Geometry: final body of the model. Coordinates: model frame, mm. Face numbers are marked on the shaded views. A direction names the side the tool comes from. Give positions to 0.01 mm unless a question says otherwise; leave off trailing zeros. Order: outer loops, then holes, each group sorted by start corner. A loop starts at its lowest first (then second) coordinate and runs counter-clockwise, first axis right, second up. Notation, with made-up numbers: (23, 53) -> (60, 53) arc R14 ccw to (60, 73) -> close; hole circle Ø5 at (18.25, 19). An arc over 180 degrees is marked (long way). Write item = value, one per line.
```python
from build123d import *

# Parameters (mm, degrees)
SKETCH1_W                      = 55
SKETCH1_H                      = 55
BOSS_EXTRUDE1_DEPTH            = 6.35
SKETCH2_W                      = 11.25
SKETCH2_H                      = 11.25
CUT_EXTRUDE1_DEPTH             = 7.35
SKETCH3_W                      = 14
SKETCH3_H                      = 8.5
CUT_EXTRUDE2_DEPTH             = 2
CBORE_FOR_M2_SHCS2_D           = 2.4
CBORE_FOR_M2_SHCS2_DEPTH       = 6.35
CBORE_FOR_M2_SHCS2_CBORE_D     = 4.4
CBORE_FOR_M2_SHCS2_CBORE_DEPTH = 2
SKETCH6_R                      = 3.25
BOSS_EXTRUDE2_DEPTH            = 5
CBORE_FOR_M2_SHCS1_D           = 2.4
CBORE_FOR_M2_SHCS1_CBORE_D     = 4.4
CBORE_FOR_M2_SHCS1_CBORE_DEPTH = 2
SKETCH13_R                     = 3.025
CUT_EXTRUDE4_DEPTH             = 1
CHAMFER1_SIZE                  = 2
SKETCH16_W                     = 10
SKETCH16_H                     = 10
BOSS_EXTRUDE3_DEPTH            = 6.35
SKETCH17_R                     = 2.55
CUT_EXTRUDE6_DEPTH             = 12.35
FILLET1_R                      = 5
FILLET2_R                      = 1
SKETCH18_R                     = 2.25
CUT_EXTRUDE7_DEPTH             = 1


with BuildPart() as part:
    # Sketch1 → Boss-Extrude1 (new body)
    with BuildSketch(Plane(origin=(0, 0, 0), x_dir=(1, 0, 0), z_dir=(0, 1, 0))):
        Rectangle(SKETCH1_W, SKETCH1_H)
    extrude(amount=BOSS_EXTRUDE1_DEPTH)

    # Sketch2 → Cut-Extrude1 (cut, through all)
    with BuildSketch(Plane(origin=(0, 6.35, 0), x_dir=(1, 0, 0), z_dir=(0, 1, 0))):
        Rectangle(SKETCH2_W, SKETCH2_H)
    extrude(amount=-CUT_EXTRUDE1_DEPTH, mode=Mode.SUBTRACT)

    # Sketch3 → Cut-Extrude2 (cut)
    with BuildSketch(Plane(origin=(0, 6.35, 0), x_dir=(1, 0, 0), z_dir=(0, 1, 0))):
        with Locations((0, -9.875)):
            Rectangle(SKETCH3_W, SKETCH3_H)
    extrude(amount=-CUT_EXTRUDE2_DEPTH, mode=Mode.SUBTRACT)

    # CBORE for M2 SHCS2
    with Locations(Plane.XZ):
        with Locations((10.5, -0.1), (10.5, 12.4), (-10.5, 12.4), (-10.5, -0.1)):
            CounterBoreHole(CBORE_FOR_M2_SHCS2_D / 2, CBORE_FOR_M2_SHCS2_CBORE_D / 2, CBORE_FOR_M2_SHCS2_CBORE_DEPTH, depth=CBORE_FOR_M2_SHCS2_DEPTH)

    # Sketch6 → Boss-Extrude2 (add)
    with BuildSketch(Plane(origin=(0, 6.35, 0), x_dir=(1, 0, 0), z_dir=(0, 1, 0))):
        with Locations((-20, 20)):
            Circle(SKETCH6_R)
        with Locations((20, 20)):
            Circle(SKETCH6_R)
        with Locations((20, -20)):
            Circle(SKETCH6_R)
        with Locations((-20, -20)):
            Circle(SKETCH6_R)
    extrude(amount=BOSS_EXTRUDE2_DEPTH)

    # CBORE for M2 SHCS1 (through all)
    with Locations(Plane.XZ):
        with Locations((-20, -20), (-20, 20), (20, 20), (20, -20)):
            CounterBoreHole(CBORE_FOR_M2_SHCS1_D / 2, CBORE_FOR_M2_SHCS1_CBORE_D / 2, CBORE_FOR_M2_SHCS1_CBORE_DEPTH)

    # Sketch13 → Cut-Extrude4 (cut)
    with BuildSketch(Plane(origin=(0, 6.35, 0), x_dir=(1, 0, 0), z_dir=(0, 1, 0))):
        with Locations((-10.5, -12.4)):
            Circle(SKETCH13_R)
        with Locations((-10.5, 0.1)):
            Circle(SKETCH13_R)
        with Locations((10.5, -12.4)):
            Circle(SKETCH13_R)
        with Locations((10.5, 0.1)):
            Circle(SKETCH13_R)
    extrude(amount=-CUT_EXTRUDE4_DEPTH, mode=Mode.SUBTRACT)

    # Chamfer1
    chamfer1_edges = [part.edges().sort_by_distance(p)[0] for p in [
        (5.625, 0, 0),
        (0, 0, 5.625),
        (-5.625, 0, 0),
        (0, 0, -5.625),
    ]]
    chamfer(chamfer1_edges, length=CHAMFER1_SIZE)

    # Sketch16 → Boss-Extrude3 (add)
    with BuildSketch(Plane.XZ):
        with Locations((32.5, 0)):
            Rectangle(SKETCH16_W, SKETCH16_H)
        with Locations((-32.5, 0)):
            Rectangle(SKETCH16_W, SKETCH16_H)
    extrude(amount=-BOSS_EXTRUDE3_DEPTH)

    # Sketch17 → Cut-Extrude6 (cut, through all)
    with BuildSketch(Plane.XZ):
        with Locations((32.5, 0)):
            Circle(SKETCH17_R)
        with Locations((-32.5, 0)):
            Circle(SKETCH17_R)
    extrude(amount=-CUT_EXTRUDE6_DEPTH, mode=Mode.SUBTRACT)

    # Fillet1
    fillet1_edges = [part.edges().sort_by_distance(p)[0] for p in [
        (27.5, 3.175, 5),
        (27.5, 3.175, -5),
        (-27.5, 3.175, -5),
        (-27.5, 3.175, 5),
        (27.5, 3.175, 27.5),
        (-27.5, 3.175, 27.5),
        (-27.5, 3.175, -27.5),
        (27.5, 3.175, -27.5),
    ]]
    fillet(fillet1_edges, radius=FILLET1_R)

    # Fillet2
    fillet2_edges = [part.edges().sort_by_distance(p)[0] for p in [
        (37.5, 3.175, -5),
        (37.5, 3.175, 5),
        (-37.5, 3.175, 5),
        (-37.5, 3.175, -5),
    ]]
    fillet(fillet2_edges, radius=FILLET2_R)

    # Sketch18 → Cut-Extrude7 (cut)
    with BuildSketch(Plane(origin=(0, 11.35, 0), x_dir=(1, 0, 0), z_dir=(0, 1, 0))):
        with Locations((-20, 20)):
            Circle(SKETCH18_R)
        with Locations((-20, -20)):
            Circle(SKETCH18_R)
        with Locations((20, 20)):
            Circle(SKETCH18_R)
        with Locations((20, -20)):
            Circle(SKETCH18_R)
    extrude(amount=-CUT_EXTRUDE7_DEPTH, mode=Mode.SUBTRACT)


solid = part.part
```
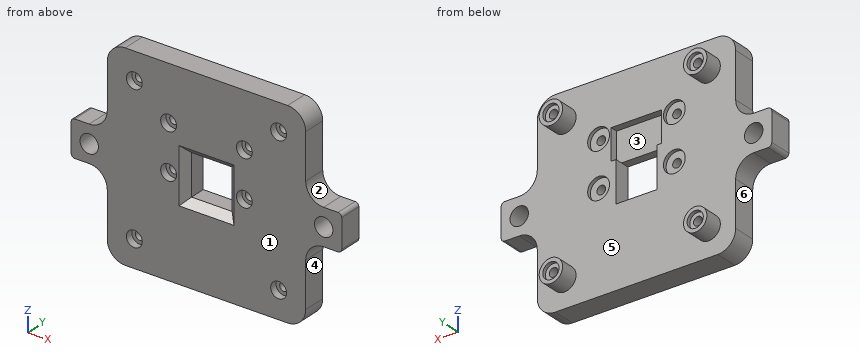
1) Reachability of the marked faces 4, 5 and 6 from +Z, -Z, +X, -X, +Y, -Y: full face, straight path, thin tool, end or side. Return the list, or none.
Check sheet entries:
face_4 = -Z, +X, +Y, -Y
face_5 = +Y
face_6 = -Z, -X, +Y, -Y
2) Section query C-C (x = 2). Output: boundary loops of the cut face in (y, z) (3 decimals).
Check sheet entries:
outline = (0, -27.5) -> (6.35, -27.5) -> (6.35, -5.625) -> (2, -5.625) -> (0, -7.625) -> close; (0, 7.625) -> (2, 5.625) -> (4.35, 5.625) -> (4.35, 14.125) -> (6.35, 14.125) -> (6.35, 27.5) -> (0, 27.5) -> close
3) Mould query, pull axis Z, two halves, no side actions, for the marked faces 1, 2 and 3. Classes: +Z half, -Z half, draft (parallel to the pull), parting line (faces both ways), or undercut.
Check sheet entries:
face_1 = draft
face_2 = +Z half
face_3 = undercut
4) Section query A-A (x = -10.5). Output: boundary loops of the cut face in (y, z) (3 decimals), plus the area to 3 significant figures.
Check sheet entries:
outline = (0, -27.5) -> (6.35, -27.5) -> (6.35, -3.125) -> (5.35, -3.125) -> (5.35, -1.3) -> (2, -1.3) -> (2, -2.3) -> (0, -2.3) -> close; (0, 2.1) -> (2, 2.1) -> (2, 1.1) -> (5.35, 1.1) -> (5.35, 2.925) -> (6.35, 2.925) -> (6.35, 9.375) -> (5.35, 9.375) -> (5.35, 11.2) -> (2, 11.2) -> (2, 10.2) -> (0, 10.2) -> close; (0, 14.6) -> (2, 14.6) -> (2, 13.6) -> (5.35, 13.6) -> (5.35, 15.425) -> (6.35, 15.425) -> (6.35, 27.5) -> (0, 27.5) -> close
area = 303 mm²
5) Section query D-D (z = 20). Count the separate pieces of the cut face and the enclosed holes in it, plus the area to 3 significant figures.
Check sheet entries:
separate_pieces = 3
enclosed_holes = 0
area = 348 mm²
6) Line query: line 1 (Z direction, x = 10.5, y = 0.6); line 2 (Z direction, x = 20, y = 0.55); line 3 (X direction, y = 6, z = 12.4) (3 decimals). Output: solid intervals per line, ascending. Write a range as from..to.
Check sheet entries:
line_1 = -27.5..-2.3, 2.1..10.2, 14.6..27.5
line_2 = -27.5..-22.2, -17.8..17.8, 22.2..27.5
line_3 = -27.5..-13.525, -7.475..-7, 7..7.475, 13.525..27.5
7) First-contact query: P1, Ø1.4, axis at x = -10.5, z = 12.4, coming from the -Y side; P2, Ø1.2, axis at x = 34, y = 2, coming from the +Z side; P3, Ø2, axis at x = -34.5, y = 2.5, coming from the -Z side; P4, Ø6, axis at x = 10.5, z = -21, coming from the +Y side. Flat tips, straight axial feed; report the tip coordinate or a pass-through.
Check sheet entries:
P1 = through
P2 = 5
P3 = -5
P4 = 6.35
8) Section query B-B (y = 9.25). Output: boundary loops of the cut face in (x, z).
Check sheet entries:
outline = circle Ø6.5 at (-20, -20); circle Ø6.5 at (-20, 20); circle Ø6.5 at (20, -20); circle Ø6.5 at (20, 20); hole circle Ø2.4 at (-20, -20); hole circle Ø2.4 at (-20, 20); hole circle Ø2.4 at (20, -20); hole circle Ø2.4 at (20, 20)
